Can you work these out from the model? Positions are in its coordinate system, mm. A direction names the side the tool comes from. Round coordinates to 2 decimals unless told otherwise and drop trailing zeros. Loops run counter-clockwise (first coordinate to the right, second up) from the corner with the lowest first, then second, coordinate; pieces in that order, holes last. Notation, with made-up numbers: (15, 50) -> (59, 50) arc R25 cw to (59, 66) -> close; hole circle Ø11 at (-21.5, 5). An arc over 180 degrees is marked (long way). Answer as a JSON object with one key per item and string values.
```python
from build123d import *

# Parameters (mm, degrees)
SKETCH1_R               = 41.9
TOP_PART_DEPTH          = 15
SKETCH2_R               = 30
CUT_EXTRUDE1_DEPTH      = 20
FILLET1_R               = 1.5
CHAMFER1_SIZE           = 2
SKETCH8_7_R             = 1.625
CUT_EXTRUDE8_DEPTH      = 3
SKETCH8_R               = 1.625
CUT_EXTRUDE7_DEPTH      = 62.124626857
CUT_EXTRUDE11_DEPTH     = 62.124626857
SKETCH15_R              = 1.625
CUT_EXTRUDE14_DEPTH     = 10
CUT_EXTRUDE15_DEPTH     = 10
CIRPATTERN1_COUNT       = 4
CIRPATTERN2_COUNT       = 4
SKETCH3_R               = 41.9
BOTTOM_PART_DEPTH       = 20
SKETCH6_R               = 37.9
CUT_EXTRUDE3_DEPTH      = 63.076324134
SKETCH_1_W              = 43
SKETCH_1_H              = 43
EXTRUDE_1_DEPTH         = 8
FILLET_1_R              = 5
CUT_EXTRUDE4_DEPTH      = 63.076324134
CUT_EXTRUDE4_DEPTH_BACK = 63.076324134
SKETCH7_R               = 17.5
SKETCH7_R_2             = 1
SKETCH12_W              = 39.5
SKETCH12_H              = 39.5
CUT_EXTRUDE10_DEPTH     = 8.5
FILLET3_R               = 2
SKETCH17_R              = 1.625
CUT_EXTRUDE16_DEPTH     = 63.076324134
SKETCH18_R              = 3
CUT_EXTRUDE17_DEPTH     = 63.076324134
SKETCH19_R              = 2.75
BOSS_EXTRUDE1_DEPTH     = 18.5
SKETCH20_W              = 87.79908129
SKETCH20_H              = 93.09964502
CUT_EXTRUDE18_DEPTH     = 10
SKETCH21_W              = 20
SKETCH21_H              = 8.651798588
CUT_EXTRUDE19_DEPTH     = 15
SKETCH23_R              = 30
CUT_EXTRUDE21_DEPTH     = 65.313451299
SKETCH24_R              = 41.9
CUT_EXTRUDE22_DEPTH     = 10


with BuildPart() as part:
    # Sketch1 → Top-Part (new body)
    with BuildSketch(Plane(origin=(0, 0, 0), x_dir=(1, 0, 0), z_dir=(0, 1, 0))):
        with Locations(Location((0, 0, 0), (0, 0, 270))):
            Circle(SKETCH1_R)
    extrude(amount=TOP_PART_DEPTH)

    # Sketch2 → Cut-Extrude1 (cut)
    with BuildSketch(Plane(origin=(0, 15, 0), x_dir=(1, 0, 0), z_dir=(0, 1, 0))):
        with Locations(Location((0, 0, 0), (0, 0, 270))):
            Circle(SKETCH2_R)
    extrude(amount=-CUT_EXTRUDE1_DEPTH, mode=Mode.SUBTRACT)

    # Fillet1
    fillet1_edges = [part.edges().sort_by_distance(p)[0] for p in [
        (0, 15, -41.9),
    ]]
    fillet(fillet1_edges, radius=FILLET1_R)

    # Chamfer1
    chamfer1_edges = [part.edges().sort_by_distance(p)[0] for p in [
        (0, 15, -30),
    ]]
    chamfer(chamfer1_edges, length=CHAMFER1_SIZE)

    # Sketch8<7> → Cut-Extrude8 (cut)
    # profile 1 of 4: a face of its own
    with BuildSketch(Plane(origin=(0, 15, 0), x_dir=(1, 0, 0), z_dir=(0, 1, 0))):
        Polygon((25.083213555, 22.516777398), (28.056316743, 23.598898462), (28.605724005, 26.714741882), (26.182028081, 28.748464238), (23.208924893, 27.666343174), (22.659517631, 24.550499754), align=None)
        with Locations(Location((25.632620818, 25.632620818, 0), (0, 0, 270))):
            Circle(SKETCH8_7_R, mode=Mode.SUBTRACT)
    # profile 2 of 4: a face of its own
    with BuildSketch(Plane(origin=(0, 15, 0), x_dir=(1, 0, 0), z_dir=(0, 1, 0))):
        Polygon((-22.516777398, 25.083213555), (-23.598898462, 28.056316743), (-26.714741882, 28.605724005), (-28.748464238, 26.182028081), (-27.666343174, 23.208924893), (-24.550499754, 22.659517631), align=None)
        with Locations(Location((-25.632620818, 25.632620818, 0), (0, 0, 270))):
            Circle(SKETCH8_7_R, mode=Mode.SUBTRACT)
    # profile 3 of 4: a face of its own
    with BuildSketch(Plane(origin=(0, 15, 0), x_dir=(1, 0, 0), z_dir=(0, 1, 0))):
        Polygon((22.516777398, -25.083213555), (23.598898462, -28.056316743), (26.714741882, -28.605724005), (28.748464238, -26.182028081), (27.666343174, -23.208924893), (24.550499754, -22.659517631), align=None)
        with Locations(Location((25.632620818, -25.632620818, 0), (0, 0, 270))):
            Circle(SKETCH8_7_R, mode=Mode.SUBTRACT)
    # profile 4 of 4: a face of its own
    with BuildSketch(Plane(origin=(0, 15, 0), x_dir=(1, 0, 0), z_dir=(0, 1, 0))):
        Polygon((-25.083213555, -22.516777398), (-28.056316743, -23.598898462), (-28.605724005, -26.714741882), (-26.182028081, -28.748464238), (-23.208924893, -27.666343174), (-22.659517631, -24.550499754), align=None)
        with Locations(Location((-25.632620818, -25.632620818, 0), (0, 0, 270))):
            Circle(SKETCH8_7_R, mode=Mode.SUBTRACT)
    extrude(amount=-CUT_EXTRUDE8_DEPTH, mode=Mode.SUBTRACT)

    # Sketch8 → Cut-Extrude7 (cut, through all)
    with BuildSketch(Plane(origin=(0, 15, 0), x_dir=(1, 0, 0), z_dir=(0, 1, 0))):
        with Locations(Location((-25.632620818, 25.632620818, 0), (0, 0, 270))):
            Circle(SKETCH8_R)
        with Locations(Location((25.632620818, 25.632620818, 0), (0, 0, 270))):
            Circle(SKETCH8_R)
        with Locations(Location((25.632620818, -25.632620818, 0), (0, 0, 270))):
            Circle(SKETCH8_R)
        with Locations(Location((-25.632620818, -25.632620818, 0), (0, 0, 270))):
            Circle(SKETCH8_R)
    extrude(amount=-CUT_EXTRUDE7_DEPTH, mode=Mode.SUBTRACT)

    # Sketch13 → Cut-Extrude11 (cut, through all)
    with BuildSketch(Plane.XZ):
        with BuildLine():
            Line((-10, 35.519149765), (-10, 40.689187753))
            ThreePointArc((-10, 40.689187753), (0, 41.9), (10, 40.689187753))
            Line((10, 40.689187753), (10, 35.519149765))
            ThreePointArc((10, 35.519149765), (0, 36.9), (-10, 35.519149765))
        make_face()
    extrude(amount=-CUT_EXTRUDE11_DEPTH, mode=Mode.SUBTRACT)

    # Sketch15 → Cut-Extrude14 (cut, symmetric)
    with BuildSketch(Plane.XY.offset(32.4)):
        with Locations(Location((0, 7.5, 0), (0, 0, 180))):
            Circle(SKETCH15_R)
    cut_extrude14 = extrude(amount=CUT_EXTRUDE14_DEPTH, both=True, mode=Mode.SUBTRACT)

    # Sketch16 → Cut-Extrude15 (cut)
    with BuildSketch(Plane.XY.offset(32.4)):
        Polygon((3.377499075, 7.5), (1.688749537, 10.425), (-1.688749537, 10.425), (-3.377499075, 7.5), (-1.688749537, 4.575), (1.688749537, 4.575), align=None)
    cut_extrude15 = extrude(amount=-CUT_EXTRUDE15_DEPTH, mode=Mode.SUBTRACT)

    # CirPattern1: Cut-Extrude14 ×4 about axis
    cirpattern1_axis = Axis((0, 0, 0), (0, 1, 0))
    for i in range(1, CIRPATTERN1_COUNT):
        add(cut_extrude14.rotate(cirpattern1_axis, i * 360 / CIRPATTERN1_COUNT), mode=Mode.SUBTRACT)

    # CirPattern2: Cut-Extrude15 ×4 about axis
    cirpattern2_axis = Axis((0, 0, 0), (0, 1, 0))
    for i in range(1, CIRPATTERN2_COUNT):
        add(cut_extrude15.rotate(cirpattern2_axis, i * 360 / CIRPATTERN2_COUNT), mode=Mode.SUBTRACT)

    # Sketch21 → Cut-Extrude19 (cut)
    with BuildSketch(Plane(origin=(0, 15, 0), x_dir=(1, 0, 0), z_dir=(0, 1, 0))):
        with Locations((0, -39.225899294)):
            Rectangle(SKETCH21_W, SKETCH21_H)
    extrude(amount=-CUT_EXTRUDE19_DEPTH, mode=Mode.SUBTRACT)


with BuildPart() as body_2:
    # Sketch3 → Bottom-Part (new body)
    with BuildSketch(Plane.XZ):
        with Locations(Location((0, 0, 0), (0, 0, 270))):
            Circle(SKETCH3_R)
    extrude(amount=BOTTOM_PART_DEPTH)

    # Sketch6 → Cut-Extrude3 (cut, through all)
    with BuildSketch(Plane(origin=(0, -1.5, 0), x_dir=(1, 0, 0), z_dir=(0, 1, 0))):
        with Locations(Location((0, 0, 0), (0, 0, 270))):
            Circle(SKETCH6_R)
    extrude(amount=-CUT_EXTRUDE3_DEPTH, mode=Mode.SUBTRACT)

    # ｽｹｯﾁ1 → ﾎﾞｽ - 押し出し1 (add)
    with BuildSketch(Plane(origin=(0, 0, 0), x_dir=(1, 0, 0), z_dir=(0, 1, 0))):
        Rectangle(SKETCH_1_W, SKETCH_1_H)
    extrude(amount=EXTRUDE_1_DEPTH)

    # ﾌｨﾚｯﾄ1
    fillet_1_edges = [body_2.edges().sort_by_distance(p)[0] for p in [
        (-21.5, 4, -21.5),
        (-21.5, 4, 21.5),
        (21.5, 4, 21.5),
        (21.5, 4, -21.5),
    ]]
    fillet(fillet_1_edges, radius=FILLET_1_R)

    # Sketch7 → Cut-Extrude4 (cut, two sides: drawn at the far end of the back side and taken through both)
    with BuildSketch(Plane(origin=(0, -1.5, 0), x_dir=(1, 0, 0), z_dir=(0, 1, 0)).offset(-CUT_EXTRUDE4_DEPTH_BACK)):
        with Locations(Location((0, 0, 0), (0, 0, 270))):
            Circle(SKETCH7_R)
        with Locations(Location((17, -17, 0), (0, 0, 270))):
            Circle(SKETCH7_R_2)
        with Locations(Location((-17, -17, 0), (0, 0, 270))):
            Circle(SKETCH7_R_2)
        with Locations(Location((-17, 17, 0), (0, 0, 270))):
            Circle(SKETCH7_R_2)
        with Locations(Location((17, 17, 0), (0, 0, 270))):
            Circle(SKETCH7_R_2)
    extrude(amount=CUT_EXTRUDE4_DEPTH + CUT_EXTRUDE4_DEPTH_BACK, mode=Mode.SUBTRACT)

    # Sketch12 → Cut-Extrude10 (cut)
    with BuildSketch(Plane.XZ.offset(1.5)):
        Rectangle(SKETCH12_W, SKETCH12_H)
    extrude(amount=-CUT_EXTRUDE10_DEPTH, mode=Mode.SUBTRACT)

    # Fillet3
    fillet3_edges = [body_2.edges().sort_by_distance(p)[0] for p in [
        (-19.75, 2.75, -19.75),
        (-19.75, 2.75, 19.75),
        (19.75, 2.75, 19.75),
        (19.75, 2.75, -19.75),
    ]]
    fillet(fillet3_edges, radius=FILLET3_R)

    # Sketch17 → Cut-Extrude16 (cut, through all)
    with BuildSketch(Plane.XZ.offset(1.5)):
        with Locations(Location((25.632620818, -25.632620818, 0), (0, 0, 90))):
            Circle(SKETCH17_R)
        with Locations(Location((-25.632620818, -25.632620818, 0), (0, 0, 90))):
            Circle(SKETCH17_R)
        with Locations(Location((25.632620818, 25.632620818, 0), (0, 0, 90))):
            Circle(SKETCH17_R)
        with Locations(Location((-25.632620818, 25.632620818, 0), (0, 0, 90))):
            Circle(SKETCH17_R)
    extrude(amount=-CUT_EXTRUDE16_DEPTH, mode=Mode.SUBTRACT)

    # Sketch18 → Cut-Extrude17 (cut, through all)
    with BuildSketch(Plane.XZ.offset(1.5)):
        with Locations((-25.632620818, 25.632620818)):
            Circle(SKETCH18_R)
        with Locations((25.632620818, 25.632620818)):
            Circle(SKETCH18_R)
        with Locations((25.632620818, -25.632620818)):
            Circle(SKETCH18_R)
        with Locations((-25.632620818, -25.632620818)):
            Circle(SKETCH18_R)
    extrude(amount=CUT_EXTRUDE17_DEPTH, mode=Mode.SUBTRACT)

    # Sketch19 → Boss-Extrude1 (add)
    # profile 1 of 4: a face of its own
    with BuildSketch(Plane.XZ.offset(1.5)):
        with BuildLine():
            Line((-6, 33), (-6, 37.422052322))
            ThreePointArc((-6, 37.422052322), (0, 37.9), (6, 37.422052322))
            Line((6, 37.422052322), (6, 33))
            ThreePointArc((6, 33), (0, 27), (-6, 33))
        make_face()
        with Locations(Location((0, 33, 0), (0, 0, 270))):
            Circle(SKETCH19_R, mode=Mode.SUBTRACT)
    # profile 2 of 4: a face of its own
    with BuildSketch(Plane.XZ.offset(1.5)):
        with BuildLine():
            Line((33, 6), (37.422052322, 6))
            ThreePointArc((37.422052322, 6), (37.9, 0), (37.422052322, -6))
            Line((37.422052322, -6), (33, -6))
            ThreePointArc((33, -6), (27, 0), (33, 6))
        make_face()
        with Locations(Location((33, 0, 0), (0, 0, 270))):
            Circle(SKETCH19_R, mode=Mode.SUBTRACT)
    # profile 3 of 4: a face of its own
    with BuildSketch(Plane.XZ.offset(1.5)):
        with BuildLine():
            Line((6, -33), (6, -37.422052322))
            ThreePointArc((6, -37.422052322), (0, -37.9), (-6, -37.422052322))
            Line((-6, -37.422052322), (-6, -33))
            ThreePointArc((-6, -33), (0, -27), (6, -33))
        make_face()
        with Locations(Location((0, -33, 0), (0, 0, 270))):
            Circle(SKETCH19_R, mode=Mode.SUBTRACT)
    # profile 4 of 4: a face of its own
    with BuildSketch(Plane.XZ.offset(1.5)):
        with BuildLine():
            Line((-33, -6), (-37.422052322, -6))
            ThreePointArc((-37.422052322, -6), (-37.9, 0), (-37.422052322, 6))
            Line((-37.422052322, 6), (-33, 6))
            ThreePointArc((-33, 6), (-27, 0), (-33, -6))
        make_face()
        with Locations(Location((-33, 0, 0), (0, 0, 270))):
            Circle(SKETCH19_R, mode=Mode.SUBTRACT)
    extrude(amount=BOSS_EXTRUDE1_DEPTH)

    # Sketch20 → Cut-Extrude18 (cut)
    with BuildSketch(Plane.XZ.offset(20)):
        Rectangle(SKETCH20_W, SKETCH20_H)
    extrude(amount=-CUT_EXTRUDE18_DEPTH, mode=Mode.SUBTRACT)

    # Sketch23 → Cut-Extrude21 (cut, through all)
    with BuildSketch(Plane(origin=(0, 15, 0), x_dir=(1, 0, 0), z_dir=(0, 1, 0))):
        with Locations(Location((0, 0, 0), (0, 0, 270))):
            Circle(SKETCH23_R)
    extrude(amount=-CUT_EXTRUDE21_DEPTH, mode=Mode.SUBTRACT)

    # Sketch24 → Cut-Extrude22 (cut)
    with BuildSketch(Plane.XZ.offset(10)):
        Circle(SKETCH24_R)
    extrude(amount=-CUT_EXTRUDE22_DEPTH, mode=Mode.SUBTRACT)


solid = part.part
```
Q1. I want a section at C-C, the plane y = 1. Write out the boundary of the cut face in (x, z) (3 decimals).
Determined:
{"outline": "(-10, 34.9) -> (-10, 40.689) arc R41.9 ccw (long way) to (10, 40.689) -> (10, 34.9) -> close; hole circle Ø60 at (0, 0); hole circle Ø3.25 at (-25.633, -25.633); hole circle Ø3.25 at (-25.633, 25.633); hole circle Ø3.25 at (25.633, -25.633); hole circle Ø3.25 at (25.633, 25.633)"}
Q2. I'm going to push flat-ended pins straight in: pin 1 (3 mm diameter, centred on x = -0.5, y = 2.5, fed in from -Z); pin 2 (3 mm diameter, centred on x = 0, y = 7.5, fed in from -Z); pin 3 (6.5 mm diameter, centred on y = 4, z = 38.5, fed in from -X); pin 4 (5 mm diameter, centred on x = 0, y = 7.5, fed in from +Z). Where does each tip first touch, or does it pass through?
Determined:
{"pin 1": "z = -41.9", "pin 2": "through", "pin 3": "x = -22.65", "pin 4": "z = 34.9"}
Q3. We'd pull the mould along Z, two halves only. Please class faces 3 (the flat face through (0, 4.575, 31)), 4 (the flat face through (-31.123, 8.942, 2.545)): pulls with the +Z half, pulls with the -Z half, needs draft (parallel to the pull), parting line crosses it, or undercut.
Determined:
{"face 3": "undercut", "face 4": "undercut"}
Q4. If I drill on L1, parallel to X at y = 9.25, z = 25; L2, parallel to Y at x = 32.5, z = 0 (3 decimals); L3, parallel to Z at x = 15, y = 6.75, over which ranges is the centre line in solid material (lowest first)? Write a range as [from, to].
Determined:
{"L1": "[-33.62, -27.13], [-24.14, -16.58], [16.58, 24.14], [27.13, 33.62]", "L2": "[0, 5.875], [9.125, 15]", "L3": "[-39.12, -25.98], [25.98, 39.12]"}
Q5. On a 3-axis mill with a long thin cutter (end or side, diameter ignored), from which of +Z, -Z, +X, -X, +Y, -Y can I reach the whole of each face in a straight line? I mean faces 1 (the flat face through (-24, 12, -24)), 2 (the flat face through (0, 4.575, -31)). Say none if no direction works.
Determined:
{"face 1": "+Y", "face 2": "none"}
Q6. I want a section at B-B, the plane z = 0. Write out the boundary of the cut face in (x, y) (3 decimals), then the cut area to 3 significant figures.
Determined:
{"outline": "(-41.9, 0) -> (-30, 0) -> (-30, 4.575) -> (-32.4, 4.575) -> (-32.4, 5.875) -> (-41.9, 5.875) -> close; (-41.9, 9.125) -> (-32.4, 9.125) -> (-32.4, 10.425) -> (-30, 10.425) -> (-30, 13) -> (-32, 15) -> (-40.4, 15) arc R1.5 ccw to (-41.9, 13.5) -> close; (30, 0) -> (41.9, 0) -> (41.9, 5.875) -> (32.4, 5.875) -> (32.4, 4.575) -> (30, 4.575) -> close; (30, 10.425) -> (32.4, 10.425) -> (32.4, 9.125) -> (41.9, 9.125) -> (41.9, 13.5) arc R1.5 ccw to (40.4, 15) -> (32, 15) -> (30, 13) -> close", "area": "262 mm²"}
Q7. I want a section at A-A, the plane x = 0. Write out the boundary of the cut face in (y, z) (3 decimals), then the cut area to 3 significant figures.
Determined:
{"outline": "(0, -41.9) -> (5.875, -41.9) -> (5.875, -32.4) -> (4.575, -32.4) -> (4.575, -30) -> (0, -30) -> close; (0, 30) -> (4.575, 30) -> (4.575, 32.4) -> (5.875, 32.4) -> (5.875, 34.9) -> (0, 34.9) -> close; (9.125, -41.9) -> (13.5, -41.9) arc R1.5 ccw to (15, -40.4) -> (15, -32) -> (13, -30) -> (10.425, -30) -> (10.425, -32.4) -> (9.125, -32.4) -> close; (9.125, 32.4) -> (10.425, 32.4) -> (10.425, 30) -> (13, 30) -> (15, 32) -> (15, 34.9) -> (9.125, 34.9) -> close", "area": "180 mm²"}
